Source: CAD feature listing. Evaluate the final solid. Frame: model axes, mm. Face numbers are marked on the shaded views. A direction names the side the tool comes from. Give positions to 0.01 mm unless a question says otherwise; leave off trailing zeros. Write each loop counter-clockwise with the first axis right and the second up, starting at its lowest first coordinate (ties: lowest second). Pieces come first, ordered by that corner, then holes. Notation, with made-up numbers: M 36,-28 L 70,-28 A33 ccw 70,4 Z; hole C -33.5,-6 d6. An arc over 180 degrees is marked long. Return JSON: item names as keys, results as strings.
```python
from build123d import *

# Parameters (mm, degrees)
BOSS_EXTRUDE1_DEPTH   = 47.0789
BOSS_EXTRUDE2_DEPTH   = 2.54
F_6_CLEARANCE_HOLE1_D = 3.7973
CUT_EXTRUDE1_DEPTH    = 87.844214731
FILLET1_R             = 2.54
F_6_CLEARANCE_HOLE2_D = 3.7973
BOSS_EXTRUDE3_DEPTH   = 38.00094


with BuildPart() as part:
    # Sketch1 → Boss-Extrude1 (new body)
    with BuildSketch(Plane.XY):
        Polygon((-59.2709, 1.778), (-59.2709, 6.35), (-46.5709, 6.35), (-46.5709, 44.35094), (-26.7589, 44.35094), (-26.7589, 39.77894), (-41.9989, 39.77894), (-41.9989, 6.35), (-41.9989, 1.778), (-46.5709, 1.778), align=None)
    extrude(amount=BOSS_EXTRUDE1_DEPTH)

    # Sketch2 → Boss-Extrude2 (add)
    with BuildSketch(Plane.XY.offset(47.0789)):
        Polygon((-26.7589, 39.77894), (-41.9989, 29.11094), (-41.9989, 39.77894), align=None)
    boss_extrude2 = extrude(amount=-BOSS_EXTRUDE2_DEPTH)

    # Mirror1: Boss-Extrude2 across plane
    add(boss_extrude2.mirror(Plane(origin=(0, 0, 23.53945), x_dir=(1, 0, 0), z_dir=(0, 0, -1))))

    # #6 Clearance Hole1 (through all)
    with Locations(Plane(origin=(0, 44.35094, 0), x_dir=(1, 0, 0), z_dir=(0, 1, 0))):
        with Locations((-36.4998, -8.0391), (-36.4998, -39.0398)):
            Hole(F_6_CLEARANCE_HOLE1_D / 2)

    # Sketch5 → Cut-Extrude1 (cut, through all)
    with BuildSketch(Plane(origin=(0, 44.35094, 0), x_dir=(1, 0, 0), z_dir=(0, 1, 0))):
        with BuildLine():
            Line((-26.7589, -23.53945), (-26.7589, -14.213831785))
            ThreePointArc((-26.7589, -14.213831785), (-31.96082, -23.53945), (-26.7589, -32.865068215))
            Line((-26.7589, -32.865068215), (-26.7589, -23.53945))
        make_face()
    extrude(amount=-CUT_EXTRUDE1_DEPTH, mode=Mode.SUBTRACT)

    # Fillet1
    fillet1_edges = [part.edges().sort_by_distance(p)[0] for p in [
        (-46.5709, 25.35047, 0),
        (-46.5709, 25.35047, 47.0789),
        (-26.7589, 42.06494, 47.0789),
        (-26.7589, 42.06494, 0),
    ]]
    fillet(fillet1_edges, radius=FILLET1_R)

    # #6 Clearance Hole2 (through all)
    with Locations(Plane(origin=(0, 6.35, 0), x_dir=(1, 0, 0), z_dir=(0, 1, 0))):
        with Locations((-52.9209, -10.83945), (-52.9209, -36.23945)):
            Hole(F_6_CLEARANCE_HOLE2_D / 2)

    # Sketch8 → Boss-Extrude3 (add)
    with BuildSketch(Plane.XZ.offset(-39.77894)):
        Polygon((-41.9989, 44.5389), (-41.9989, 39.0398), (-36.4998, 44.5389), align=None)
        Polygon((-41.9989, 2.54), (-36.4998, 2.54), (-41.9989, 8.0391), align=None)
    extrude(amount=BOSS_EXTRUDE3_DEPTH)


solid = part.part
```
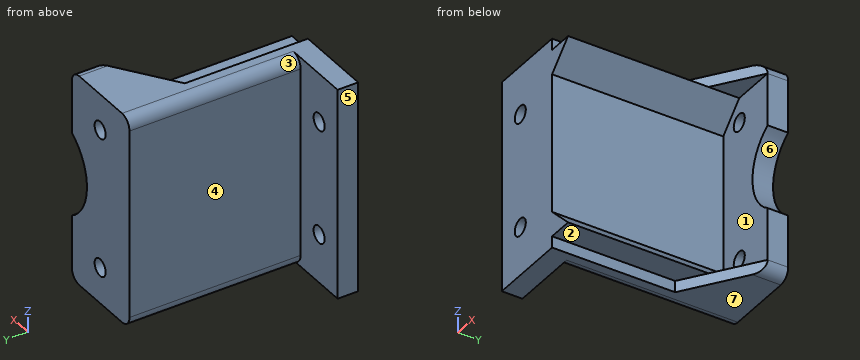
1) Cut plane A-A, the plane y = 15.5. Return the cut outline in (x, z), then the cut area to 3 significant figures.
Numbers:
{"outline": "M -46.57,2.54 A2.54 ccw -44.03,0 L -42,0 L -42,2.54 L -36.5,2.54 L -42,8.04 L -42,39.04 L -36.5,44.54 L -42,44.54 L -42,47.08 L -44.03,47.08 A2.54 ccw -46.57,44.54 Z", "area": "243 mm²"}
2) Set-up query: the marked faces 1, 2, 3 and 4. Return all of +Z, -Z, +X, -X, +Y, -Y with unobstructed straight access to the full face (end or side cutting, diameter ignored); none if empty.
Numbers:
{"face 1": "+X, -Y", "face 2": "-Z, +X, -Y", "face 3": "+Z, -X, +Y", "face 4": "+Z, -Z, -X, +Y"}
3) Contact query for flat-ended pins moving along their axis: pin 1 Ø8 at (x, z) = (-31, 20.5) entering from -Y; pin 2 Ø2 at (x, z) = (-50, 12.5) entering from +Y; pin 3 Ø9.5 at (y, z) = (19, 23) entering from +X; pin 4 Ø2.5 at (x, z) = (-36.5, 8.04) entering from +Y. Output: stop coordinate, or through.
Numbers:
{"pin 1": "stops at y = 39.78", "pin 2": "stops at y = 6.35", "pin 3": "stops at x = -42", "pin 4": "passes through"}
4) Draft query along Z for the marked faces 5, 6 and 7. Return one class per face: released by +Z, released by -Z, zero draft, split by the parting line, or undercut.
Numbers:
{"face 5": "zero draft", "face 6": "undercut", "face 7": "released by -Z"}
5) Cut plane C-C, the plane z = 22. Return the cut outline in (x, y).
Numbers:
{"outline": "M -59.27,1.78 L -42,1.78 L -42,39.78 L -31.85,39.78 L -31.85,44.35 L -46.57,44.35 L -46.57,6.35 L -59.27,6.35 Z"}
6) Cut plane D-D, the plane z = 15. Return the cut outline in (x, y), then the cut area to 3 significant figures.
Numbers:
{"outline": "M -59.27,1.78 L -42,1.78 L -42,39.78 L -27.87,39.78 L -27.87,44.35 L -46.57,44.35 L -46.57,6.35 L -59.27,6.35 Z", "area": "317 mm²"}
7) Line query: line 1 (Y direction, x = -51, z = 43); line 2 (Y direction, x = -34, z = 20); line 3 (Z direction, x = -29.5, y = 38). Output: solid intervals per line, ascending. Write a range as [from, to].
Numbers:
{"line 1": "y = [1.78, 6.35]", "line 2": "y = [39.78, 44.35]", "line 3": "z = [0, 2.54], [44.54, 47.08]"}
8) Cut plane B-B, the plane x = -41. Return the cut outline in (y, z), then the cut area to 3 significant figures.
Numbers:
{"outline": "M 1.78,2.54 L 29.81,2.54 L 29.81,0 L 44.35,0 L 44.35,47.08 L 29.81,47.08 L 29.81,44.54 L 1.78,44.54 L 1.78,40.04 L 39.78,40.04 L 39.78,7.04 L 1.78,7.04 Z", "area": "608 mm²"}
